Check sheet for the drawn part. Datum: minimum x, y, z corner. Units: mm. Coordinates: 2 decimals unless noted, no trailing zeros. Loops run counter-clockwise (first coordinate to the right, second up) from the corner with the lowest first, then second, coordinate; pieces in that order, holes last.
Q1. Sectioned sample at B-B (x = 27). Enter the section's corners in (y, z) (1 decimal).
Q2. Material ranges on probe 1 along Z at (x, y) = (4, 0.6); probe 2 along X at (y, z) = (1.35, 33.5) (1 decimal); probe 3 along X at (y, z) = (0.1, 35) (1 decimal), recorded low to high.
Q3. Sectioned sample at C-C (y = 0.9). Enter the section's corners in (x, z) (1 decimal).
Q4. Sectioned sample at A-A (z = 10). Enter the section's corners in (x, y).
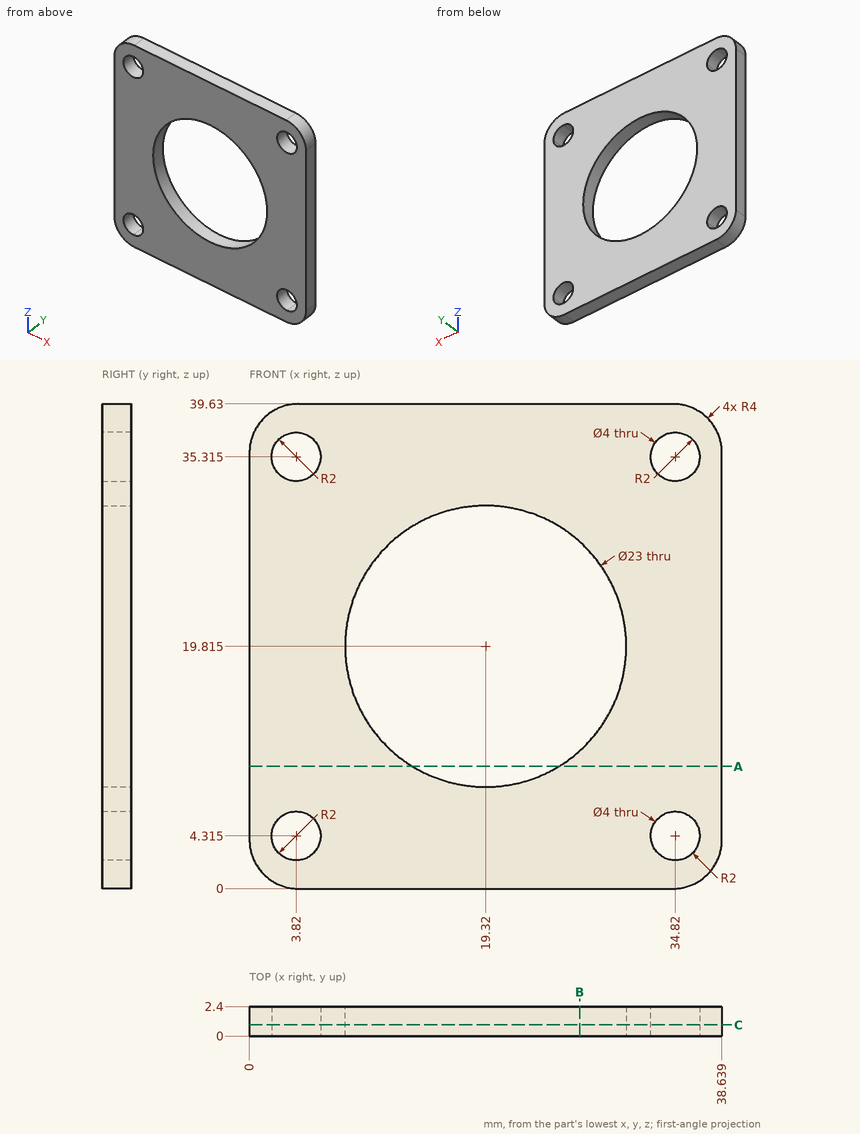
Geometry check:
1. outline: (0, 0) - (2.4, 0) - (2.4, 11.3) - (0, 11.3) - close; (0, 28.4) - (2.4, 28.4) - (2.4, 39.6) - (0, 39.6) - close
2. probe 1: z = 0 to 2.32, 6.31 to 33.32, 37.31 to 39.63
2. probe 2: x = 0 to 3, 4.7 to 34, 35.7 to 38.6
2. probe 3: x = 0 to 1.8, 5.8 to 32.8, 36.8 to 38.6
3. outline: (0, 4) arc R4 ccw to (4, 0) - (34.6, 0) arc R4 ccw to (38.6, 4) - (38.6, 35.6) arc R4 ccw to (34.6, 39.6) - (4, 39.6) arc R4 ccw to (0, 35.6) - close; hole circle Ø4 at (3.8, 4.3); hole circle Ø4 at (3.8, 35.3); hole circle Ø23 at (19.3, 19.8); hole circle Ø4 at (34.8, 4.3); hole circle Ø4 at (34.8, 35.3)
4. outline: (0, 0) - (13.33, 0) - (13.33, 2.4) - (0, 2.4) - close; (25.31, 0) - (38.64, 0) - (38.64, 2.4) - (25.31, 2.4) - close
